Read the model definition and answer for the solid it produces. Units are mm, in the model's axes. A direction names the side the tool comes from. Round coordinates to 2 decimals unless told otherwise and drop trailing zeros. Order: outer loops, then holes, each group sorted by start corner. A loop starts at its lowest first (then second) coordinate and runs counter-clockwise, first axis right, second up. Notation, with made-up numbers: M -15,70.5 L 35,70.5 A8 ccw 35,80.5 Z; hole C 11,65.25 d2. An arc over 180 degrees is marked long. Use one line per item in the form item = value. Start each with the question number.
from build123d import *

# Parameters (mm, degrees)
SKETCH2_R           = 3.5
BOSS_EXTRUDE1_DEPTH = 10
SKETCH4_R           = 119
SKETCH3_R           = 104


with BuildPart() as part:
    # Sketch2 → Boss-Extrude1 (new body)
    with BuildSketch(Plane(origin=(0, 0, 0), x_dir=(1, 0, 0), z_dir=(0, 1, 0))):
        with BuildLine():
            Line((-94, 104), (94, 104))
            ThreePointArc((94, 104), (101.071067812, 101.071067812), (104, 94))
            Line((104, 94), (104, -94))
            ThreePointArc((104, -94), (101.071067812, -101.071067812), (94, -104))
            Line((94, -104), (-94, -104))
            ThreePointArc((-94, -104), (-101.071067812, -101.071067812), (-104, -94))
            Line((-104, -94), (-104, 94))
            ThreePointArc((-104, 94), (-101.071067812, 101.071067812), (-94, 104))
        make_face()
        with Locations(Location((-89, 89, 0), (0, 0, 270))):
            Circle(SKETCH2_R, mode=Mode.SUBTRACT)
        with Locations(Location((89, 89, 0), (0, 0, 270))):
            Circle(SKETCH2_R, mode=Mode.SUBTRACT)
        with Locations(Location((89, -89, 0), (0, 0, 270))):
            Circle(SKETCH2_R, mode=Mode.SUBTRACT)
        with Locations(Location((-89, -89, 0), (0, 0, 270))):
            Circle(SKETCH2_R, mode=Mode.SUBTRACT)
    extrude(amount=BOSS_EXTRUDE1_DEPTH)

    # Sketch4 → Loft1 section 0
    with BuildSketch(Plane(origin=(0, 220, 0), x_dir=(1, 0, 0), z_dir=(0, 1, 0))):
        Circle(SKETCH4_R)
    # Sketch3 → Loft1 section 1
    with BuildSketch(Plane(origin=(0, 10, 0), x_dir=(1, 0, 0), z_dir=(0, 1, 0))):
        Circle(SKETCH3_R)
    loft()


solid = part.part
Item 1: Section D-D (y = 90) is taken. Write down the section's boundary in (x, z), and give its area (3 significant figures).
Item 2: For a pull along Y with two mould halves and no side action, classify faces 1 (the flat face through (-2, 220, -2)), 2 (the flat face through (104, 5, -1)), 3 (the flat face through (-79, 10, -83)), 4 (the flat face through (-79, 10, 83)) as pulls with the +Y half, pulls with the -Y half, needs draft (parallel to the pull), parting line crosses it, or undercut.
Item 3: Find the intervals of material crossed by L1, parallel to X at y = 4, z = 89; L2, parallel to Z at x = -65.5, y = 61.5; L3, parallel to Z at x = 90, y = 160, in increasing order. Write a range as [from, to].
Item 4: Section B-B (x = -89) is taken. Give the number of separate pieces and of enclosed holes in the cut face, and give its area (3 significant figures).
Item 5: Section A-A (y = 55.5) is taken. Write down the section's boundary in (x, z).
Item 6: Given P1, Ø2, axis at x = 87, z = 11.5, coming from the -Y side; P2, Ø6, axis at x = 88, y = 157, coming from the +Z side; P3, Ø3, axis at y = 47.5, z = 4.5, coming from the -X side; P4, Ø1, axis at x = -84.5, y = 172, coming from the +Z side, each flat-ended and moving along its own axis, determine where each tip first touches the part or whether it passes through.
Item 7: A tool of negligible diameter and unlimited length cuts with its end or side. For faces 5 (the flat face through (1, 5, 104)), 6 (the flat face through (-104, 5, 1)), 7 (the conical face through (-24.148, 113.53, 108.746)), from which of +Z, -Z, +X, -X, +Y, -Y can it reach the whole face along a straight path? Write none if from no direction.
The answers:
q1.outline = C 0,0 d219.43
q1.area = 37,800 mm²
q2.face_1 = pulls with the +Y half
q2.face_2 = needs draft
q2.face_3 = undercut
q2.face_4 = undercut
q3.L1 = [-104, -92.5], [-85.5, 85.5], [92.5, 104]
q3.L2 = [-85.47, 85.47]
q3.L3 = [-71.13, 71.13]
q4.separate_pieces = 3
q4.enclosed_holes = 0
q4.area = 30,000 mm²
q5.outline = C 0,0 d214.5
q6.P1 = 0
q6.P2 = 76.73
q6.P3 = -106.71
q6.P4 = 79.38
q7.face_5 = +Z, +X, -X, -Y
q7.face_6 = +Z, -Z, -X, -Y
q7.face_7 = none
